Build history of the part. All positions in model axes, mm. Face numbers are marked on the shaded views. A direction names the side the tool comes from. Round coordinates to 2 decimals unless told otherwise and drop trailing zeros. Loops run counter-clockwise (first coordinate to the right, second up) from the corner with the lowest first, then second, coordinate; pieces in that order, holes last. Notation, with made-up numbers: M 54,-3 L 108,-3 A23 cw 108,33 Z; hole C 7.25,69.25 d7. An arc over 180 degrees is marked long. One line per item, written item: value.
```python
from build123d import *

# Parameters (mm, degrees)
BASPROSKE_W                    = 5
BASPROSKE_H                    = 15.75
TOOTHCUT_DEPTH                 = 23.828162432
TEETHCUTS_COUNT                = 16
TEETHCUTS_ANGLE                = 337.5
BORSKE_R                       = 3.5
BORE_DEPTH                     = 50.0000508
M2_CLEARANCE_HOLE1_D           = 2.2
M2_CLEARANCE_HOLE1_CSINK_D     = 2.25
M2_CLEARANCE_HOLE1_CSINK_ANGLE = 90


with BuildPart() as part:
    # BasProSke → Base-Revolve (revolve)
    with BuildSketch(Plane(origin=(0, 0, 0), x_dir=(1, 0, 0), z_dir=(0, 1, 0)), mode=Mode.PRIVATE) as base_revolve_sk:
        with Locations((2.5, 7.875)):
            Rectangle(BASPROSKE_W, BASPROSKE_H)
    revolve(base_revolve_sk.sketch.rotate(Axis((-10, 0, 0), (1, 0, 0)), 180), axis=Axis((-10, 0, 0), (1, 0, 0)))

    # TooCutSke → ToothCut (cut, through all)
    with BuildSketch(Plane(origin=(0, 0, 0), x_dir=(0, 0, -1), z_dir=(1, 0, 0))):
        with BuildLine():
            ThreePointArc((0.896728289, 11.777411032), (0, 11.8115), (-0.896728289, 11.777411032))
            ThreePointArc((-0.896728289, 11.777411032), (-1.421809307, 13.833768969), (-2.674397607, 15.547052537))
            ThreePointArc((-2.674397607, 15.547052537), (0, 15.7754), (2.674397607, 15.547052537))
            ThreePointArc((2.674397607, 15.547052537), (1.421809307, 13.833768969), (0.896728289, 11.777411032))
        make_face()
    toothcut = extrude(amount=TOOTHCUT_DEPTH, mode=Mode.SUBTRACT)

    # TeethCuts: ToothCut ×16 about axis
    teethcuts_axis = Axis((-10, 0, 0), (1, 0, 0))
    for i in range(1, TEETHCUTS_COUNT):
        add(toothcut.rotate(teethcuts_axis, i * TEETHCUTS_ANGLE / (TEETHCUTS_COUNT - 1)), mode=Mode.SUBTRACT)

    # BorSke → Bore (cut, symmetric)
    with BuildSketch(Plane(origin=(0, 0, 0), x_dir=(0, 0, -1), z_dir=(1, 0, 0))):
        with Locations(Location((0, 0, 0), (0, 0, 180))):
            Circle(BORSKE_R)
    extrude(amount=BORE_DEPTH, both=True, mode=Mode.SUBTRACT)

    # M2 Clearance Hole1 (through all)
    with Locations(Plane(origin=(5, 0, 0), x_dir=(0, 0, -1), z_dir=(1, 0, 0))):
        with Locations((-5.055813485, 5.055813485), (5.055813485, 5.055813485), (5.055813485, -5.055813485), (-5.055813485, -5.055813485)):
            CounterSinkHole(M2_CLEARANCE_HOLE1_D / 2, M2_CLEARANCE_HOLE1_CSINK_D / 2, counter_sink_angle=M2_CLEARANCE_HOLE1_CSINK_ANGLE)


solid = part.part
```
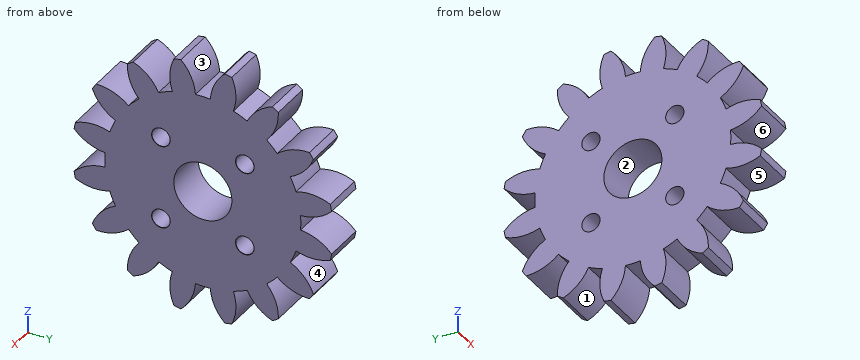
Item 1: Wall check: line 1 along Z through (x, y) = (2.2, 8); line 2 along Z through (x, y) = (0.65, -8.5); line 3 along Y through (x, z) = (2.3, -5). Give the ranges that are in metal, low to high.
Check values:
line 1: z = -13.16 to -9.34, -8.69 to 8.69, 9.34 to 13.16
line 2: z = -13.26 to -10.15, -8.2 to 8.2, 10.15 to 13.26
line 3: y = -10.7 to -6.15, -3.96 to 3.96, 6.15 to 10.7
Item 2: Drop flat-ended pins along their axis: P1, Ø3, axis at x = 2.5, y = 11, coming from the -Z side; P2, Ø1.8, axis at y = 5.06, z = 5.06, coming from the +X side; P3, Ø1.5, axis at x = 4.5, z = -9, coming from the +Y side. Give the stop position or say it passes through.
Check values:
P1: stops at z = -9.1
P2: passes through
P3: stops at y = 13.33
Item 3: Slice it at A-A, the plane z = 0. Give the cut face in (x, y), and give its area (3 significant figures).
Check values:
outline: M 0,-11.81 L 5,-11.81 L 5,-3.5 L 0,-3.5 Z; M 0,3.5 L 5,3.5 L 5,11.81 L 0,11.81 Z
area: 83.1 mm2
Item 4: Which spindle directions (+Z, -Z, +X, -X, +Y, -Y) get a long thin tool onto all of the face, cutting with end or side? Do the marked faces 4, 5 and 6. Say none if no direction does.
Check values:
face 4: +X, -X, +Y
face 5: +X, -X
face 6: +X, -X, -Y
Item 5: Pull direction Z, two halves, no side cores. Call the marked faces 1, 2 and 3: pulls with the +Z half, pulls with the -Z half, needs draft (parallel to the pull), parting line crosses it, or undercut.
Check values:
face 1: pulls with the -Z half
face 2: undercut
face 3: pulls with the +Z half
Item 6: Slice it at D-D, the plane z = 10. Give the cut face in (x, y), and give its area (3 significant figures).
Check values:
outline: M 0,-8.42 L 5,-8.42 L 5,8.42 L 0,8.42 Z
area: 84.2 mm2
Item 7: Slice it at C-C, the plane x = 2.75. Give the number of separate pieces and of enclosed holes in the cut face, and give its area (3 significant figures).
Check values:
separate pieces: 1
enclosed holes: 5
area: 536 mm2
